Part model, mm, in its own coordinate system. Face numbers are marked on the shaded views. A direction names the side the tool comes from. Coordinates: 2 decimals unless noted, no trailing zeros. Loops run counter-clockwise (first coordinate to the right, second up) from the corner with the lowest first, then second, coordinate; pieces in that order, holes last. Notation, with made-up numbers: M 17,85 L 50,85 A22 cw 50,124 Z; hole C -12.75,15.5 d11. An arc over 180 degrees is marked long. Use a Markdown table: item, result. Add a question column.
1) Band-saw the part on C-C (y = 63.5). List the corners of the cut face in (x, z) (3 decimals).
2) Band-saw the part on D-D (z = -52). List the corners of the cut face in (x, y) (3 decimals), plus the area to 3 significant figures.
3) Band-saw the part on A-A (z = -35.5). List the corners of the cut face in (x, y) (3 decimals).
4) Pin check, flat tips, straight feed: pin 1 Ø2.5 at (y, z) = (-131.5, -46) entering from +X (3 decimals); pin 2 Ø9 at (x, y) = (117.475, 117.475) entering from -Z; pin 3 Ø3.5 at (y, z) = (-131.5, -51) entering from -X (3 decimals). Stop position of each tip, or through.
5) Tool access for the marked faces 1 and 2: list every direction of +Z, -Z, +X, -X, +Y, -Y with a clear straight run to the whole face (end or side of a thin tool).
6) Wall check: probe 1 along Y at (x, z) = (-11.5, -47) (3 decimals); probe 2 along Z at (x, y) = (19, 67). Give the ranges that are in metal, low to high. Write a range as from..to.
7) Band-saw the part on B-B (x = -90.5). List the corners of the cut face in (y, z) (1 decimal), plus the area to 3 significant figures.
from build123d import *

# Parameters (mm, degrees)
SKETCH1_W                      = 260.35
SKETCH1_H                      = 260.35
BASE_FLANGE1_DEPTH             = 3.2639
EDGE_FLANGE1_STRIP_W           = 18.36928
EDGE_FLANGE1_STRIP_H           = 3.2639
EDGE_FLANGE1_STRIP_CUT_DEPTH   = 260.35
EDGE_FLANGE1_STRIP_2_W         = 18.36928
EDGE_FLANGE1_STRIP_2_H         = 3.2639
EDGE_FLANGE1_STRIP_CUT_2_DEPTH = 260.35
EDGE_FLANGE1_DEPTH             = 260.35
EDGE_FLANGE1_BEND_DEPTH        = 260.35
SKETCH16_W                     = 13.208
SKETCH16_H                     = 63.5
CUT_EXTRUDE1_DEPTH             = 307.55461301
CUT_EXTRUDE2_DEPTH             = 307.55461301
FILLET1_R                      = 12.7
F_10_0_1935_DIAMETER_HOLE1_D   = 4.9149
FILLET2_R                      = 1.27
F_1_4_CLEARANCE_HOLE1_D        = 6.7564


# Sheet-metal steps are written as plain solids
with BuildPart() as part:
    # Sketch1 → Base-Flange1 (new body)
    with BuildSketch(Plane.XY):
        Rectangle(SKETCH1_W, SKETCH1_H)
    extrude(amount=-BASE_FLANGE1_DEPTH)

    # Edge-Flange1 strip (across the edge) → Edge-Flange1 strip cut (cut)
    with BuildSketch(Plane(origin=(-130.175, 130.175, -3.2639), x_dir=(0, -1, 0), z_dir=(1, 0, 0))):
        with Locations((-6.5278, -1.63195)):
            Rectangle(EDGE_FLANGE1_STRIP_W, EDGE_FLANGE1_STRIP_H)
    extrude(amount=EDGE_FLANGE1_STRIP_CUT_DEPTH, mode=Mode.SUBTRACT)

    # Edge-Flange1 strip 2 (across the edge) → Edge-Flange1 strip cut 2 (cut)
    with BuildSketch(Plane(origin=(130.175, -130.175, -3.2639), x_dir=(0, 1, 0), z_dir=(-1, 0, 0))):
        with Locations((-6.5278, -1.63195)):
            Rectangle(EDGE_FLANGE1_STRIP_2_W, EDGE_FLANGE1_STRIP_2_H)
    extrude(amount=EDGE_FLANGE1_STRIP_CUT_2_DEPTH, mode=Mode.SUBTRACT)

    # Edge-Flange1 section (across the edge) → Edge-Flange1 (add)
    with BuildSketch(Plane(origin=(-130.175, 130.175, -3.2639), x_dir=(0, -1, 0), z_dir=(1, 0, 0))):
        with BuildLine():
            Line((-3.2639, 2.65684), (-3.2639, 72.9361))
            Line((-3.2639, 72.9361), (0, 72.9361))
            Line((0, 72.9361), (0, 2.65684))
            ThreePointArc((0, 2.65684), (0.778170419, 0.778170419), (2.65684, 0))
            Line((2.65684, 0), (2.65684, -3.2639))
            ThreePointArc((2.65684, -3.2639), (-1.529755404, -1.529755404), (-3.2639, 2.65684))
        make_face()
    extrude(amount=EDGE_FLANGE1_DEPTH)

    # Edge-Flange1 section 2 (across the edge) → Edge-Flange1 bend (add)
    with BuildSketch(Plane(origin=(130.175, -130.175, -3.2639), x_dir=(0, 1, 0), z_dir=(-1, 0, 0))):
        with BuildLine():
            Line((-3.2639, 2.65684), (-3.2639, 72.9361))
            Line((-3.2639, 72.9361), (0, 72.9361))
            Line((0, 72.9361), (0, 2.65684))
            ThreePointArc((0, 2.65684), (0.778170419, 0.778170419), (2.65684, 0))
            Line((2.65684, 0), (2.65684, -3.2639))
            ThreePointArc((2.65684, -3.2639), (-1.529755404, -1.529755404), (-3.2639, 2.65684))
        make_face()
    extrude(amount=EDGE_FLANGE1_BEND_DEPTH)

    # Sketch16 → Cut-Extrude1 (cut, through all)
    with BuildSketch(Plane(origin=(0, 133.4389, 0), x_dir=(1, 0, 0), z_dir=(0, 1, 0))):
        with Locations((0, 44.45)):
            Rectangle(SKETCH16_W, SKETCH16_H)
    extrude(amount=-CUT_EXTRUDE1_DEPTH, mode=Mode.SUBTRACT)

    # Sketch18 → Cut-Extrude2 (cut, through all)
    with BuildSketch(Plane(origin=(0, 133.4389, 0), x_dir=(1, 0, 0), z_dir=(0, 1, 0))):
        Polygon((-130.175, 76.2), (-130.175, 25.4), (-28.575, 76.2), align=None)
        Polygon((130.175, 76.2), (28.575, 76.2), (130.175, 25.4), align=None)
    extrude(amount=-CUT_EXTRUDE2_DEPTH, mode=Mode.SUBTRACT)

    # Fillet1
    fillet1_edges = [part.edges().sort_by_distance(p)[0] for p in [
        (-28.575, 131.80695, -76.2),
        (-130.175, 131.80695, -25.4),
        (-28.575, -131.80695, -76.2),
        (-130.175, -131.80695, -25.4),
        (28.575, 131.80695, -76.2),
        (130.175, 131.80695, -25.4),
        (130.175, -131.80695, -25.4),
        (28.575, -131.80695, -76.2),
    ]]
    fillet(fillet1_edges, radius=FILLET1_R)

    # #10 (0.1935) Diameter Hole1 (through all)
    with Locations(Plane(origin=(0, 133.4389, 0), x_dir=(1, 0, 0), z_dir=(0, 1, 0))):
        with Locations((-19.304, 22.225), (-19.304, 66.675), (19.304, 66.675), (19.304, 22.225)):
            Hole(F_10_0_1935_DIAMETER_HOLE1_D / 2)

    # Fillet2
    fillet2_edges = [part.edges().sort_by_distance(p)[0] for p in [
        (-6.604, 131.80695, -76.2),
        (6.604, 131.80695, -12.7),
        (-6.604, 131.80695, -12.7),
        (6.604, 131.80695, -76.2),
        (-6.604, -131.80695, -12.7),
        (-6.604, -131.80695, -76.2),
        (6.604, -131.80695, -76.2),
        (6.604, -131.80695, -12.7),
    ]]
    fillet(fillet2_edges, radius=FILLET2_R)

    # 1/4 Clearance Hole1 (through all)
    with Locations(Plane.XY):
        with Locations((117.475, 117.475), (-117.475, -117.475), (-117.475, 117.475), (117.475, -117.475)):
            Hole(F_1_4_CLEARANCE_HOLE1_D / 2)


solid = part.part
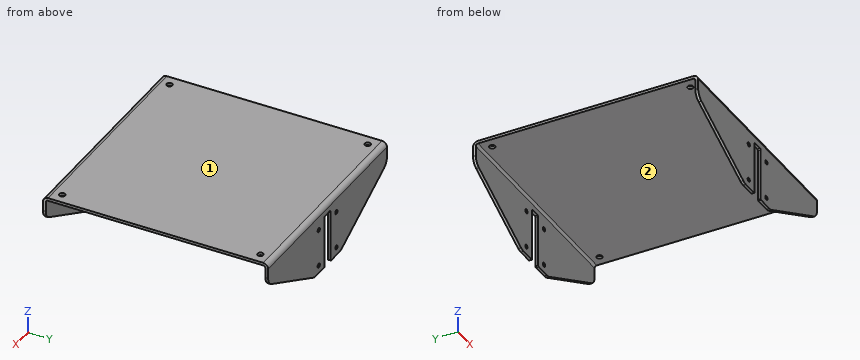
Entries:
| question | item | result |
|---|---|---|
| 1 | outline | M -130.175,-3.264 L 130.175,-3.264 L 130.175,0 L -130.175,0 Z |
| 2 | outline | M -76.975,-133.439 L -6.604,-133.439 L -6.604,-130.175 L -76.975,-130.175 Z; M -76.975,130.175 L -6.604,130.175 L -6.604,133.439 L -76.975,133.439 Z; M 6.604,-133.439 L 76.975,-133.439 L 76.975,-130.175 L 6.604,-130.175 Z; M 6.604,130.175 L 76.975,130.175 L 76.975,133.439 L 6.604,133.439 Z |
| 2 | area | 919 mm2 |
| 3 | outline | M -109.975,-133.439 L -6.604,-133.439 L -6.604,-130.175 L -109.975,-130.175 Z; M -109.975,130.175 L -6.604,130.175 L -6.604,133.439 L -109.975,133.439 Z; M 6.604,-133.439 L 109.975,-133.439 L 109.975,-130.175 L 6.604,-130.175 Z; M 6.604,130.175 L 109.975,130.175 L 109.975,133.439 L 6.604,133.439 Z |
| 4 | pin 1 | x = 91.475 |
| 4 | pin 2 | z = -3.26 |
| 4 | pin 3 | x = -82.475 |
| 5 | face 1 | +Z, +X, -X, +Y, -Y |
| 5 | face 2 | -Z, +X, -X |
| 6 | probe 1 | -133.439..-130.175, 130.175..133.439 |
| 6 | probe 2 | -3.26..0 |
| 7 | outline | M -133.4,-45.2 L -130.2,-45.2 L -130.2,-5.9 A2.7 cw -127.5,-3.3 L 127.5,-3.3 A2.7 cw 130.2,-5.9 L 130.2,-45.2 L 133.4,-45.2 L 133.4,-5.9 A5.9 ccw 127.5,0 L -127.5,0 A5.9 ccw -133.4,-5.9 Z |
| 7 | area | 1,130 mm2 |
